Part model, mm, in its own coordinate system. Face numbers are marked on the shaded views. Give positions to 0.01 mm unless a question says otherwise; leave off trailing zeros. Loops run counter-clockwise (first coordinate to the right, second up) from the corner with the lowest first, then second, coordinate; pieces in that order, holes last. Notation, with made-up numbers: (58, -0.5) -> (72, -0.5) arc R19 ccw to (72, 35.5) -> close; hole circle Ø2 at (28.25, -31.5). An arc over 180 degrees is marked (long way). Write item = value, one per line.
from build123d import *

# Parameters (mm, degrees)
F0_R     = 15.24
F2_DEPTH = 8.89
F1_R     = 3.2258
F3_DEPTH = 8.89


with BuildPart() as f2:
    # F0 (on Top) → F2 (new body, symmetric)
    with BuildSketch(Plane.XY):
        Circle(F0_R)
    extrude(amount=F2_DEPTH, both=True)

    # F1 (on face) → F3 (cut, symmetric)
    with BuildSketch(Plane.XY):
        with Locations((6.286179, 6.286179)):
            Circle(F1_R)
        with Locations((-6.286179, 6.286179)):
            Circle(F1_R)
        with Locations((6.286179, -6.286179)):
            Circle(F1_R)
        with Locations((-6.286179, -6.286179)):
            Circle(F1_R)
    extrude(amount=F3_DEPTH, both=True, mode=Mode.SUBTRACT)


solid = f2.part
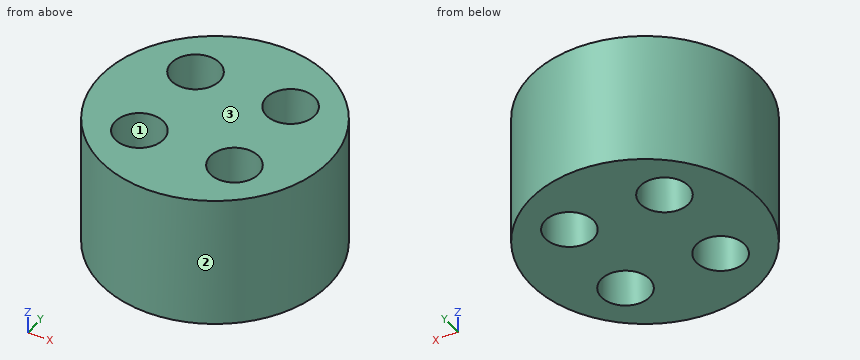
1) Slice it at C-C, the plane z = -2.5. List the corners of the cut face in (x, y), and give its area (3 significant figures).
Resolved:
outline = circle Ø30.48 at (0, 0); hole circle Ø6.45 at (-6.29, -6.29); hole circle Ø6.45 at (-6.29, 6.29); hole circle Ø6.45 at (6.29, -6.29); hole circle Ø6.45 at (6.29, 6.29)
area = 599 mm²
2) Drill centre lines: line 1 along Y through (x, z) = (-5, -2); line 2 along Y through (x, z) = (-4.5, -2.25); line 3 along X through (y, z) = (-4, 0.5). Where is each one in solid material? Low to high. Write a range as [from, to].
Resolved:
line_1 = [-14.4, -9.24], [-3.33, 3.33], [9.24, 14.4]
line_2 = [-14.56, -8.97], [-3.6, 3.6], [8.97, 14.56]
line_3 = [-14.71, -8.56], [-4.01, 4.01], [8.56, 14.71]
3) Slice it at B-B, the plane y = 4.5. List the corners of the cut face in (x, z).
Resolved:
outline = (-14.56, -8.89) -> (-8.97, -8.89) -> (-8.97, 8.89) -> (-14.56, 8.89) -> close; (-3.6, -8.89) -> (3.6, -8.89) -> (3.6, 8.89) -> (-3.6, 8.89) -> close; (8.97, -8.89) -> (14.56, -8.89) -> (14.56, 8.89) -> (8.97, 8.89) -> close
4) Slice it at A-A, the plane x = -6.5. List the corners of the cut face in (y, z), and give its area (3 significant figures).
Resolved:
outline = (-13.78, -8.89) -> (-9.5, -8.89) -> (-9.5, 8.89) -> (-13.78, 8.89) -> close; (-3.07, -8.89) -> (3.07, -8.89) -> (3.07, 8.89) -> (-3.07, 8.89) -> close; (9.5, -8.89) -> (13.78, -8.89) -> (13.78, 8.89) -> (9.5, 8.89) -> close
area = 261 mm²
5) Slice it at D-D, the plane y = -12.5. List the corners of the cut face in (x, z), and give its area (3 significant figures).
Resolved:
outline = (-8.72, -8.89) -> (8.72, -8.89) -> (8.72, 8.89) -> (-8.72, 8.89) -> close
area = 310 mm²
6) Drop flat-ended pins along their axis: P1, Ø3, axis at x = -5, z = -5.5, coming from the +Y side; P2, Ø1.5, axis at x = -5, z = 4, coming from the +Y side; P3, Ø10, axis at x = 2, z = -5.5, coming from the +Y side; P4, Ø8, axis at y = -9.5, z = 6.5, coming from the +X side. Give the stop position or say it passes through.
Resolved:
P1 = 14.83
P2 = 14.64
P3 = 15.24
P4 = 14.21
7) Pull direction X, two halves, no side cores. Call the marked faces 1, 2 and 3: pulls with the +X half, pulls with the -X half, needs draft (parallel to the pull), parting line crosses it, or undercut.
Resolved:
face_1 = undercut
face_2 = parting line crosses it
face_3 = needs draft
